Model file for the job. Use its own axes, mm. A direction names the side the tool comes from. Give positions to 0.01 mm unless a question says otherwise; leave off trailing zeros. Order: outer loops, then holes, each group sorted by start corner. A loop starts at its lowest first (then second) coordinate and runs counter-clockwise, first axis right, second up. Notation, with made-up numbers: (64, 53.5) - (123, 53.5) arc R3 cw to (123, 57.5) - close; hole circle Ø6 at (81.5, 29). An arc over 180 degrees is marked (long way). Use CSV: the item, a comma, the result in double quotes. Start each with the question number.
(1) Band-saw the part on C-C, the plane y = 17. Give the cut face in (x, z), then the cut area to 3 significant figures.
(2) Band-saw the part on B-B, the plane y = -8.5. Give the cut face in (x, z).
(3) Drop flat-ended pins along their axis: pin 1 Ø24 at (x, y) = (262.5, -7) entering from +Z; pin 2 Ø3.5 at (x, z) = (79.5, 4) entering from +Y; pin 3 Ø2 at (x, y) = (158, -28.5) entering from +Z; pin 4 Ø3.5 at (x, z) = (166, 9) entering from -Y. Give the stop position or say it passes through.
(4) Probe L1, parallel to X at y = 7, z = 16.25; L2, parallel to X at y = -11, z = 7.5; L3, parallel to Z at x = 68, y = -7.5. List the from-to ranges inside material, lowest first.
(5) Pull direction Y, two halves, no side cores. Call faces 1 (the flat face through (159, -10, 12)), 2 (the flat face through (-104, -10, 5)), 3 (the flat face through (-104, -50.64, 12)), 4 (the flat face through (159, 4.36, 6)): +Y half, -Y half, draft (parallel to the pull), parting line (faces both ways), or undercut.
(6) Tool access for faces 5 (the flat face through (-104, -45.64, 15)), 6 (the flat face through (386.973, -11, 6)), 7 (the flat face through (159, -25.64, 6)): list every direction of +Z, -Z, +X, -X, +Y, -Y with a clear straight run to the whole face (end or side of a thin tool).
(7) Band-saw the part on A-A, the plane z = 18. Give the cut face in (x, y).
(8) Band-saw the part on D-D, the plane x = 292. Give the cut face in (y, z), then the cut area to 3 significant figures.
from build123d import *

# Parameters (mm, degrees)
F0_W     = 450
F0_H     = 30
F1_DEPTH = 12
F0_W_2   = 70
F0_H_2   = 70
F2_DEPTH = 25
F3_DEPTH = 5
F5_D     = 8


with BuildPart() as f1:
    # F0 (on Top) → F1 (new body)
    with BuildSketch(Plane.XY):
        with Locations((161.972634, -10.640169)):
            Rectangle(F0_W, F0_H)
    extrude(amount=F1_DEPTH)

    # F0 (on Top) → F2 (join)
    with BuildSketch(Plane.XY):
        Polygon((-63.027366, 29.359831), (-143.027366, 29.359831), (-143.027366, -50.640169), (-63.027366, -50.640169), (-63.027366, -25.640169), (-63.027366, 4.359831), align=None)
        with Locations((-103.027366, -10.640169)):
            Rectangle(F0_W_2, F0_H_2, mode=Mode.SUBTRACT)
    extrude(amount=F2_DEPTH)

    # F0 (on Top) → F3 (join)
    with BuildSketch(Plane.XY):
        with Locations((-103.027366, -10.640169)):
            Rectangle(F0_W_2, F0_H_2)
    extrude(amount=F3_DEPTH)

    # F5 (through all)
    with Locations(Plane.XZ.offset(25.640169)):
        with Locations((186.972634, 6)):
            Hole(F5_D / 2)


solid = f1.part
Answer block:
1,outline,"(-143.03, 0) - (-63.03, 0) - (-63.03, 25) - (-68.03, 25) - (-68.03, 5) - (-138.03, 5) - (-138.03, 25) - (-143.03, 25) - close"
1,area,"600 mm2"
2,outline,"(-143.03, 0) - (386.97, 0) - (386.97, 12) - (-63.03, 12) - (-63.03, 25) - (-68.03, 25) - (-68.03, 5) - (-138.03, 5) - (-138.03, 25) - (-143.03, 25) - close; hole circle Ø8 at (186.97, 6)"
3,pin 1,"stops at z = 12"
3,pin 2,"stops at y = 4.36"
3,pin 3,"passes through"
3,pin 4,"stops at y = -25.64"
4,L1,"x = -143.03 to -138.03, -68.03 to -63.03"
4,L2,"x = -143.03 to -138.03, -68.03 to 183.26, 190.68 to 386.97"
4,L3,"z = 0 to 12"
5,face 1,"draft"
5,face 2,"undercut"
5,face 3,"-Y half"
5,face 4,"+Y half"
6,face 5,"+Z"
6,face 6,"+Z, -Z, +X, +Y, -Y"
6,face 7,"+Z, -Z, +X, -Y"
7,outline,"(-143.03, -50.64) - (-63.03, -50.64) - (-63.03, 29.36) - (-143.03, 29.36) - close; hole (-138.03, -45.64) - (-68.03, -45.64) - (-68.03, 24.36) - (-138.03, 24.36) - close"
8,outline,"(-25.64, 0) - (4.36, 0) - (4.36, 12) - (-25.64, 12) - close"
8,area,"360 mm2"
